```python
from build123d import *

# Parameters (mm, degrees)
AUFSATZ_LINEAR_AUSTRAGEN1_DEPTH = 35
VERRUNDUNG1_R                   = 1.5
FASE1_SIZE                      = 1.5


with BuildPart() as part:
    # Skizze1 → Aufsatz-Linear austragen1 (new body)
    with BuildSketch(Plane.XY):
        Polygon((-6.75, 0), (6.75, 0), (6.75, 17), (4.35, 17), (4.35, 12), (5.85, 12), (5.85, 10.5), (4.35, 10.5), (4.35, 3), (-4.35, 3), (-4.35, 10.5), (-5.85, 10.5), (-5.85, 12), (-4.35, 12), (-4.35, 17), (-6.75, 17), align=None)
    extrude(amount=AUFSATZ_LINEAR_AUSTRAGEN1_DEPTH)

    # Verrundung1
    verrundung1_edges = [part.edges().sort_by_distance(p)[0] for p in [
        (6.75, 0, 17.5),
        (-6.75, 0, 17.5),
        (-6.75, 17, 17.5),
        (-4.35, 3, 17.5),
        (4.35, 3, 17.5),
        (6.75, 17, 17.5),
    ]]
    fillet(verrundung1_edges, radius=VERRUNDUNG1_R)

    # Fase1
    fase1_edges = [part.edges().sort_by_distance(p)[0] for p in [
        (5.1, 12, 35),
        (-5.1, 12, 0),
        (-5.1, 10.5, 0),
        (5.1, 10.5, 0),
        (5.1, 12, 0),
        (5.1, 10.5, 35),
        (-5.1, 10.5, 35),
        (-5.1, 12, 35),
    ]]
    chamfer(fase1_edges, length=FASE1_SIZE)


solid = part.part
```
Input: part model. Units: mm. Frame: model coordinates. A direction names the side the tool comes from. Coordinates: 2 decimals unless noted, no trailing zeros. Loops run counter-clockwise (first coordinate to the right, second up) from the corner with the lowest first, then second, coordinate; pieces in that order, holes last.
Q1. Section B-B, the plane z = 15. Return the cut outline in (x, y).
Results are:
outline: (-6.75, 1.5) arc R1.5 ccw to (-5.25, 0) - (5.25, 0) arc R1.5 ccw to (6.75, 1.5) - (6.75, 15.5) arc R1.5 ccw to (5.25, 17) - (4.35, 17) - (4.35, 12) - (5.85, 12) - (5.85, 10.5) - (4.35, 10.5) - (4.35, 4.5) arc R1.5 cw to (2.85, 3) - (-2.85, 3) arc R1.5 cw to (-4.35, 4.5) - (-4.35, 10.5) - (-5.85, 10.5) - (-5.85, 12) - (-4.35, 12) - (-4.35, 17) - (-5.25, 17) arc R1.5 ccw to (-6.75, 15.5) - close
Q2. Set-up query: faces 1 (the flat face through (-4.35, 14, 17)), 2 (the flat face through (5, 10, 1)), 3 (the flat face through (5, 12, 17)), 4 (the flat face through (5, 10, 34)). Return all of +Z, -Z, +X, -X, +Y, -Y with unobstructed straight access to the full face (end or side cutting, diameter ignored); none if empty.
Results are:
face 1: +Z, -Z, +Y
face 2: -Z
face 3: +Z, -Z
face 4: +Z
Q3. Line query: line 1 along X through (y, z) = (13.5, 29.5); line 2 along Y through (x, z) = (4.75, 13.5); line 3 along Y through (x, z) = (3, 9). Output: solid intervals per line, ascending.
Results are:
line 1: x = -6.75 to -4.35, 4.35 to 6.75
line 2: y = 0 to 10.5, 12 to 17
line 3: y = 0 to 3.01
Q4. Section A-A, the plane y = 13. Return the cut outline in (x, z), and give its area (3 significant figures).
Results are:
outline: (-6.75, 0) - (-5.85, 0) - (-5.85, 0.5) - (-4.35, 0.5) - (-4.35, 34.5) - (-5.85, 34.5) - (-5.85, 35) - (-6.75, 35) - close; (4.35, 0.5) - (5.85, 0.5) - (5.85, 0) - (6.75, 0) - (6.75, 35) - (5.85, 35) - (5.85, 34.5) - (4.35, 34.5) - close
area: 165 mm2
Q5. Contact query for flat-ended pins moving along their axis: pin 1 (3 mm diameter, centred on x = -1, y = 14, fed in from +Z); pin 2 (1.7 mm diameter, centred on x = 0.5, z = 21, fed in from +Y); pin 3 (3 mm diameter, centred on x = 2, z = 13, fed in from +Y). Output: stop coordinate, or through.
Results are:
pin 1: passes through
pin 2: stops at y = 3
pin 3: stops at y = 3.15
Q6. Mould query, pull axis X, two halves, no side actions, for faces 5 (the cylindrical face through (-6.3, 0.43, 17.74)), 6 (the flat face through (5, 10.5, 17)), 7 (the flat face through (0, 0, 17)). Classes: +X half, -X half, draft (parallel to the pull), parting line (faces both ways), or undercut.
Results are:
face 5: -X half
face 6: undercut
face 7: draft
Q7. Section D-D, the plane x = -0.75. Return the cut outline in (y, z), and give its area (3 significant figures).
Results are:
outline: (0, 0) - (3, 0) - (3, 35) - (0, 35) - close
area: 105 mm2
Q8. Section C-C, the plane x = 3.75. Return the cut outline in (y, z).
Results are:
outline: (0, 0) - (3.3, 0) - (3.3, 35) - (0, 35) - close
